```python
from build123d import *

# Parameters (mm, degrees)
BOSS_EXTRUDE1_DEPTH = 50
SKETCH3_W           = 40
SKETCH3_H           = 2
BOSS_EXTRUDE2_DEPTH = 5
CUT_EXTRUDE1_REACH  = 62.415
SKETCH4_R           = 1.5


with BuildPart() as part:
    # Sketch1 → Boss-Extrude1 (new body)
    with BuildSketch(Plane.XY):
        Polygon((8.660254038, -15), (17.320508076, 0), (20, 0), (20, -17), (-20, -17), (-20, 0), (-17.320508076, 0), (-8.660254038, -15), align=None)
    extrude(amount=BOSS_EXTRUDE1_DEPTH)

    # Sketch3 → Boss-Extrude2 (add)
    with BuildSketch(Plane.XY.offset(50)):
        with Locations((0, -16)):
            Rectangle(SKETCH3_W, SKETCH3_H)
    boss_extrude2 = extrude(amount=BOSS_EXTRUDE2_DEPTH)

    # Sketch4 → Cut-Extrude1 (cut, up to next)
    with BuildSketch(Plane(origin=(0, -15, 0), x_dir=(1, 0, 0), z_dir=(0, 1, 0)), mode=Mode.PRIVATE) as cut_extrude1_sk1:
        with Locations(Location((0, -52.5, 0), (0, 0, 270))):
            Circle(SKETCH4_R)
    cut_extrude1_tool1 = extrude(cut_extrude1_sk1.sketch, amount=-CUT_EXTRUDE1_REACH, mode=Mode.PRIVATE) & part.part
    cut_extrude1 = cut_extrude1_tool1.solids().sort_by_distance((0, -15, 52.5))[0]
    add(cut_extrude1, mode=Mode.SUBTRACT)

    # Mirror1: Boss-Extrude2, Cut-Extrude1 across plane
    add(boss_extrude2.mirror(Plane.XY.offset(25)))
    add(cut_extrude1.mirror(Plane.XY.offset(25)), mode=Mode.SUBTRACT)


solid = part.part
```
For this review, take the finished solid that the model builds, in its own axes (mm). A direction names the side the tool comes from. Give positions to 0.01 mm unless a question says otherwise; leave off trailing zeros. Write each loop counter-clockwise with the first axis right and the second up, starting at its lowest first coordinate (ties: lowest second). Pieces come first, ordered by that corner, then holes. Notation, with made-up numbers: M 27,63.5 L 42,63.5 A22 ccw 42,91.5 Z; hole C 18,-35 d2. An arc over 180 degrees is marked long. Answer as a JSON object with one key per item and string values. Group by question number.
Item 1: Consider section A-A on z = 52.5. Write out the cut boundary in (x, y), plus the area to 3 significant figures.
Item 2: Consider section C-C on y = -8.5. Write out the cut boundary in (x, z).
Item 3: Consider section D-D on z = 7.5. Write out the cut boundary in (x, y).
Item 4: Tool access review of faces 1 (the flat face through (-13.05, -7.4, 24.65)), 2 (the flat face through (-19, 0, 25)), 3 (the flat face through (16, -9, 50)), 4 (the flat face through (-16, -9, 0)): name each direction out of +Z, -Z, +X, -X, +Y, -Y from which nothing blocks a thin tool from reaching the whole face with its end or side.
Item 5: Consider section B-B on x = 0. Write out the cut boundary in (y, z).
Item 6: For pin 1 Ø5 at (x, y) = (11, -6.5) entering from +Z; pin 2 Ø5.5 at (x, y) = (13.5, -10) entering from -Z; pin 3 Ø6 at (x, y) = (-10.5, -2.5) entering from -Z; pin 4 Ø4 at (x, z) = (0, 52.5) entering from +Y, all flat-tipped, find the tip position at first contact; note any pin that passes through.
Item 7: For probe 1 along X at (y, z) = (-15.85, -2.5); probe 2 along Z at (x, y) = (-16.5, -12.5); probe 3 along X at (y, z) = (-6.25, 32.5), list the stretches that pass through material, from the lowest coordinate up. Write a range as [from, to].
Item 8: Draft analysis for pull direction Z (two halves, no side actions). For faces 5 (the flat face through (12.93, -7.605, 24.65)), 6 (the flat face through (16, -9, 0)), 7 (the cylindrical face through (0, -16, -1)), 8 (the cylindrical face through (-0.9, -16, 51.3)), state which applies: +Z half, -Z half, draft (parallel to the pull), parting line (faces both ways), or undercut.
Check result:
{
 "1": {"outline": "M -20,-17 L -1.5,-17 L -1.5,-15 L -20,-15 Z; M 1.5,-17 L 20,-17 L 20,-15 L 1.5,-15 Z", "area": "74.0 mm^2"},
 "2": {"outline": "M -20,0 L -12.41,0 L -12.41,50 L -20,50 Z; M 12.41,0 L 20,0 L 20,50 L 12.41,50 Z"},
 "3": {"outline": "M -20,-17 L 20,-17 L 20,0 L 17.32,0 L 8.66,-15 L -8.66,-15 L -17.32,0 L -20,0 Z"},
 "4": {"face 1": "+Z, -Z, +Y", "face 2": "+Z, -Z, +X, -X, +Y", "face 3": "+Z, +X, -X, +Y", "face 4": "-Z, +X, -X, +Y"},
 "5": {"outline": "M -17,-5 L -15,-5 L -15,-4 L -17,-4 Z; M -17,-1 L -15,-1 L -15,51 L -17,51 Z; M -17,54 L -15,54 L -15,55 L -17,55 Z"},
 "6": {"pin 1": "stops at z = 50", "pin 2": "stops at z = 0", "pin 3": "passes through", "pin 4": "stops at y = -15"},
 "7": {"probe 1": "x = [-20, -1.5], [1.5, 20]", "probe 2": "z = [0, 50]", "probe 3": "x = [-20, -13.71], [13.71, 20]"},
 "8": {"face 5": "draft", "face 6": "-Z half", "face 7": "undercut", "face 8": "undercut"}
}
